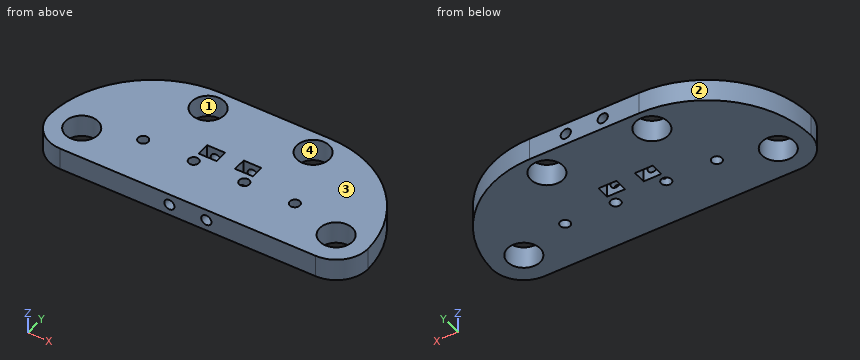
```python
from build123d import *

# Parameters (mm, degrees)
ESBO_O1_W                = 100.3
ESBO_O1_H                = 42.3
ESBO_O1_R                = 5.15
ESBO_O1_R_2              = 1.6
ESBO_O1_W_2              = 5.6
ESBO_O1_H_2              = 4.1
RESSALTO_EXTRUS_O1_DEPTH = 7
FILETE1_R                = 10
ESBO_O4_R                = 1.6
CORTE_EXTRUS_O3_DEPTH    = 67.046091306
FILETE3_R                = 33


with BuildPart() as part:
    # Esboço1 → Ressalto-extrusão1 (new body)
    with BuildSketch(Plane.XY):
        with Locations((0.087398189, -10.441132561)):
            Rectangle(ESBO_O1_W, ESBO_O1_H)
        with Locations((-16.508590221, 3.558867439)):
            Circle(ESBO_O1_R, mode=Mode.SUBTRACT)
        with Locations((16.491409779, 3.558867439)):
            Circle(ESBO_O1_R, mode=Mode.SUBTRACT)
        with Locations((-39.912601811, -21.441132561)):
            Circle(ESBO_O1_R, mode=Mode.SUBTRACT)
        with Locations((40.087398189, -21.441132561)):
            Circle(ESBO_O1_R, mode=Mode.SUBTRACT)
        with Locations((8.037398189, -16.591132561)):
            Circle(ESBO_O1_R_2, mode=Mode.SUBTRACT)
        with Locations((23.937398189, -16.591132561)):
            Circle(ESBO_O1_R_2, mode=Mode.SUBTRACT)
        with Locations((-7.862601811, -16.591132561)):
            Circle(ESBO_O1_R_2, mode=Mode.SUBTRACT)
        with Locations((-23.762601811, -16.591132561)):
            Circle(ESBO_O1_R_2, mode=Mode.SUBTRACT)
        with Locations((-5.635596016, -11.291132561)):
            Rectangle(ESBO_O1_W_2, ESBO_O1_H_2, mode=Mode.SUBTRACT)
        with Locations((5.810392394, -11.291132561)):
            Rectangle(ESBO_O1_W_2, ESBO_O1_H_2, mode=Mode.SUBTRACT)
    extrude(amount=RESSALTO_EXTRUS_O1_DEPTH)

    # Filete1
    filete1_edges = [part.edges().sort_by_distance(p)[0] for p in [
        (50.237398189, -31.591132561, 3.5),
        (-50.062601811, -31.591132561, 3.5),
    ]]
    fillet(filete1_edges, radius=FILETE1_R)

    # Esboço4 → Corte-extrusão3 (cut, through all)
    with BuildSketch(Plane(origin=(0, 10.708867439, 0), x_dir=(1, 0, 0), z_dir=(0, 1, 0))):
        with Locations(Location((-5.722601811, -3.5, 0), (0, 0, 270))):
            Circle(ESBO_O4_R)
        with Locations(Location((5.897398189, -3.5, 0), (0, 0, 270))):
            Circle(ESBO_O4_R)
    extrude(amount=-CORTE_EXTRUS_O3_DEPTH, mode=Mode.SUBTRACT)

    # Filete3
    # the kernel refuses this fillet: 33 mm, written as the material it takes off along each edge
    with BuildSketch(Plane(origin=(50.237398189, 10.708867439, -82.481437306), x_dir=(0, -1, 0), z_dir=(0, 0, 1))) as filete3_piece_1:
        with BuildLine():
            CenterArc((33, -32.992574922), FILETE3_R, 91.215456182, 88.784543818)
            Line((0, -32.992574922), (0, 0))
            Line((0, 0), (32.3, 0))
        make_face()
    extrude(amount=171.962874611, mode=Mode.SUBTRACT)
    with BuildSketch(Plane(origin=(-50.062601811, 10.708867439, -82.481437306), x_dir=(0, -1, 0), z_dir=(0, 0, 1))) as filete3_piece_2:
        with BuildLine():
            CenterArc((33, 32.992574922), FILETE3_R, 180, 88.784543818)
            Line((0, 32.992574922), (0, 0))
            Line((0, 0), (32.3, 0))
        make_face()
    extrude(amount=171.962874611, mode=Mode.SUBTRACT)


solid = part.part
```
The model under review builds one solid part; all positions refer to its coordinate system, in mm. Face numbers are marked on the shaded views. Coordinates: 2 decimals unless noted, no trailing zeros. Write each loop counter-clockwise with the first axis right and the second up, starting at its lowest first coordinate (ties: lowest second). Pieces come first, ordered by that corner, then holes.
1) We need section B-B on y = 7. State the section outline as (x, z) points, then the cut area to 3 significant figures.
2) The part is to be moulded in two halves that separate along Y. For the marked faces 1, 2, 3 and 4, say which applies: pulls with the +Y half, pulls with the -Y half, needs draft (parallel to the pull), parting line crosses it, or undercut.
3) We need section D-D on x = -38. State the section outline as (y, z) points.
4) To check wall thickness, follow probe 1 along X at (y, z) = (-24, 3.5); probe 2 along Z at (x, y) = (6, -14.5); probe 3 along X at (y, z) = (1.5, 1.75). State the ranges of each line that lie inside material, in increasing order.
5) Clearance check with flat-ended pins moving along their axes: pin 1 Ø1.9 at (x, z) = (5.9, 3.5) entering from -Y; pin 2 Ø2 at (y, z) = (-11.5, 2) entering from -X; pin 3 Ø2 at (y, z) = (-1, 5.5) entering from +X; pin 4 Ø3.5 at (y, z) = (-11, 4) entering from +X. State where each tip first meets the part, or that it passes through.
6) We need section C-C on z = 3.5. Count the separate pieces of the cut face and the enclosed holes in it, then the cut area to 3 significant figures.
7) We need section A-A on x = 41.5. State the section outline as (y, z) points.
Answer list:
1. outline: (-32.27, 0) - (-20.34, 0) - (-20.34, 7) - (-32.27, 7) - close; (-12.68, 0) - (12.66, 0) - (12.66, 7) - (-12.68, 7) - close; (20.32, 0) - (32.44, 0) - (32.44, 7) - (20.32, 7) - close; hole circle Ø3.2 at (-5.72, 3.5); hole circle Ø3.2 at (5.9, 3.5)
1. area: 330 mm2
2. face 1: undercut
2. face 2: pulls with the +Y half
2. face 3: needs draft
2. face 4: undercut
3. outline: (-31.59, 0) - (-26.22, 0) - (-26.22, 7) - (-31.59, 7) - close; (-16.66, 0) - (3.22, 0) - (3.22, 7) - (-16.66, 7) - close
4. probe 1: x = -49.77 to -44.38, -35.44 to -7.32, -4.12 to 4.3, 7.5 to 35.62, 44.56 to 49.94
4. probe 2: z = 0 to 1.9, 5.1 to 7
4. probe 3: x = -39.94 to -21.23, -11.79 to 11.77, 21.21 to 40.11
5. pin 1: passes through
5. pin 2: stops at x = -48.58
5. pin 3: stops at x = 43.27
5. pin 4: stops at x = 48.84
6. separate pieces: 3
6. enclosed holes: 6
6. area: 3,080 mm2
7. outline: (-31.51, 0) - (-26.39, 0) - (-26.39, 7) - (-31.51, 7) - close; (-16.49, 0) - (0.08, 0) - (0.08, 7) - (-16.49, 7) - close
